from build123d import *

# Parameters (mm, degrees)
LID_DEPTH             = 8
SKETCH2_R             = 3
INSETSCREWHOLES_DEPTH = 5
SKETCH3_R             = 1.75
SCREWHOLES_DEPTH      = 444.138052318
FILLET2_R             = 10
CHAMFER1_SIZE         = 2


with BuildPart() as part:
    # Sketch1 → Lid (new body)
    with BuildSketch(Plane.XY):
        Polygon((-65.612006704, -435), (-65.612006704, -135), (-45.812006704, -135), (-45.812006704, -322.5), (77.087993296, -322.5), (77.087993296, -154.8), (77.087993296, -142.3), (64.587993296, -142.3), (64.587993296, -135), (84.387993296, -135), (84.387993296, -435), (64.587993296, -435), (64.587993296, -427.7), (77.087993296, -427.7), (77.087993296, -330.5), (-45.812006704, -330.5), (-45.812006704, -435), align=None)
    extrude(amount=LID_DEPTH)

    # Sketch2 → InsetScrewHoles (cut)
    with BuildSketch(Plane.XY.offset(8)):
        with Locations((80.887993296, -147.8)):
            Circle(SKETCH2_R)
        with Locations((-61.812006704, -147.8)):
            Circle(SKETCH2_R)
        with Locations((-61.812006704, -326.5)):
            Circle(SKETCH2_R)
        with Locations((80.887993296, -326.5)):
            Circle(SKETCH2_R)
        with Locations((80.887993296, -422.2)):
            Circle(SKETCH2_R)
        with Locations((-61.812006704, -422.2)):
            Circle(SKETCH2_R)
    extrude(amount=-INSETSCREWHOLES_DEPTH, mode=Mode.SUBTRACT)

    # Sketch3 → ScrewHoles (cut, through all)
    with BuildSketch(Plane.XY.offset(3)):
        with Locations((-61.812006704, -147.8)):
            Circle(SKETCH3_R)
        with Locations((80.887993296, -147.8)):
            Circle(SKETCH3_R)
        with Locations((80.887993296, -326.5)):
            Circle(SKETCH3_R)
        with Locations((-61.812006704, -326.5)):
            Circle(SKETCH3_R)
        with Locations((80.887993296, -422.2)):
            Circle(SKETCH3_R)
        with Locations((-61.812006704, -422.2)):
            Circle(SKETCH3_R)
    extrude(amount=-SCREWHOLES_DEPTH, mode=Mode.SUBTRACT)

    # Fillet2
    fillet2_edges = [part.edges().sort_by_distance(p)[0] for p in [
        (-65.612006704, -435, 4),
        (-65.612006704, -135, 4),
        (84.387993296, -135, 4),
        (84.387993296, -435, 4),
    ]]
    fillet(fillet2_edges, radius=FILLET2_R)

    # Chamfer1
    chamfer1_edges = [part.edges().sort_by_distance(p)[0] for p in [
        (77.087993296, -232.4, 0),
    ]]
    chamfer(chamfer1_edges, length=CHAMFER1_SIZE)


solid = part.part
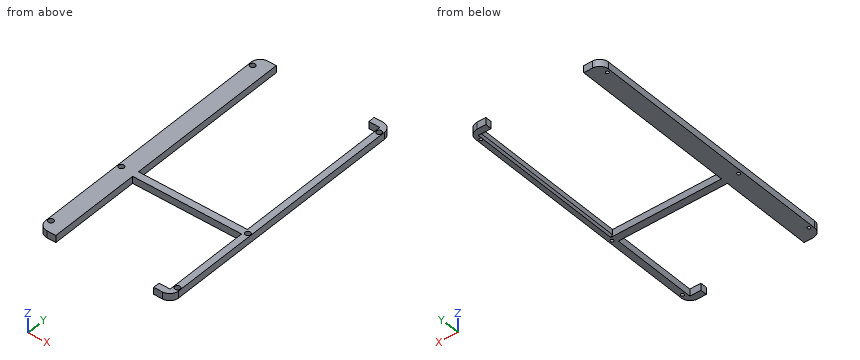
CAD build for the part. Positions are in the model's coordinates, mm. Round coordinates to 2 decimals unless told otherwise and drop trailing zeros. Write each loop counter-clockwise with the first axis right and the second up, starting at its lowest first coordinate (ties: lowest second). Pieces come first, ordered by that corner, then holes. Notation, with made-up numbers: (45, 40.5) -> (87, 40.5) arc R17 ccw to (87, 60.5) -> close; hole circle Ø6 at (65, 19). An arc over 180 degrees is marked (long way). Answer as a JSON object with one key per item and string values.
(1) Band-saw the part on C-C, the plane x = -20. List the corners of the cut face in (y, z), then the cut area to 3 significant figures.
Reported:
{"outline": "(-330.5, 0) -> (-322.5, 0) -> (-322.5, 8) -> (-330.5, 8) -> close", "area": "64.0 mm^2"}
(2) Pin check, flat tips, straight feed: P1, Ø3, axis at x = -62.5, y = -148.5, coming from the +Z side; P2, Ø1.5, axis at x = 43, z = 2, coming from the -Y side; P3, Ø3, axis at x = -61, y = -328, coming from the +Z side; P4, Ø4, axis at x = 35.5, z = 3, coming from the +Y side. Stop position of each tip, or through.
Reported:
{"P1": "stops at z = 3", "P2": "stops at y = -330.5", "P3": "stops at z = 8", "P4": "stops at y = -322.5"}
(3) Probe probe 1 along X at (y, z) = (-422.2, 6.1); probe 2 along X at (y, z) = (-214, 4.25); probe 3 along X at (y, z) = (-147.8, 2.15). List the from-to ranges inside material, lowest first. Write a range as [from, to].
Reported:
{"probe 1": "x = [-65.61, -64.81], [-58.81, -45.81], [77.09, 77.89], [83.89, 84.39]", "probe 2": "x = [-65.61, -45.81], [77.09, 84.39]", "probe 3": "x = [-65.61, -63.56], [-60.06, -45.81], [77.09, 79.14], [82.64, 84.39]"}
(4) Band-saw the part on A-A, the plane y = -360.5. List the corners of the cut face in (x, z).
Reported:
{"outline": "(-65.61, 0) -> (-45.81, 0) -> (-45.81, 8) -> (-65.61, 8) -> close; (77.09, 0) -> (84.39, 0) -> (84.39, 8) -> (77.09, 8) -> close"}
(5) Band-saw the part on B-B, the plane y = -284.5. List the corners of the cut face in (x, z), then the cut area to 3 significant figures.
Reported:
{"outline": "(-65.61, 0) -> (-45.81, 0) -> (-45.81, 8) -> (-65.61, 8) -> close; (77.09, 2) -> (79.09, 0) -> (84.39, 0) -> (84.39, 8) -> (77.09, 8) -> close", "area": "215 mm^2"}
